from build123d import *

# Parameters (mm, degrees)
BOSS_EXTRUDE1_DEPTH  = 5
SKETCH10_W           = 3
SKETCH10_H           = 3
CUT_EXTRUDE3_DEPTH   = 10
SKETCH11_W           = 10
SKETCH11_H           = 3
CUT_EXTRUDE4_DEPTH   = 10
BOSS_EXTRUDE5_DEPTH  = 3
SKETCH13_R           = 2
BOSS_EXTRUDE6_DEPTH  = 3
SKETCH14_R           = 2
SKETCH14_W           = 7
SKETCH14_H           = 3
BOSS_EXTRUDE7_DEPTH  = 3
SKETCH15_W           = 11.761480784
SKETCH15_H           = 3
BOSS_EXTRUDE8_DEPTH  = 3
SKETCH15_3_W         = 11.761480784
SKETCH15_3_H         = 3
CUT_EXTRUDE6_DEPTH   = 3
CUT_EXTRUDE7_DEPTH   = 63
BOSS_EXTRUDE9_DEPTH  = 3
BOSS_EXTRUDE10_DEPTH = 5
SKETCH19_R           = 2
CUT_EXTRUDE8_DEPTH   = 10
SKETCH24_R           = 1.75
CUT_EXTRUDE12_DEPTH  = 3
BOSS_EXTRUDE12_DEPTH = 3
CUT_EXTRUDE13_DEPTH  = 3
SKETCH27_R           = 2
CUT_EXTRUDE14_DEPTH  = 3
SKETCH29_W           = 25
SKETCH29_H           = 120
BOSS_EXTRUDE13_DEPTH = 1.4
SKETCH30_R           = 2
CUT_EXTRUDE15_DEPTH  = 30.4


with BuildPart() as part:
    # Sketch1 → Boss-Extrude1 (new body)
    with BuildSketch(Plane(origin=(0, 0, 0), x_dir=(1, 0, 0), z_dir=(0, 1, 0))):
        Polygon((-70, -55), (0, -55), (0, 55), (-70, 55), (-85, 40), (-210, 40), (-250, 0), (-210, -40), (-85, -40), align=None)
    extrude(amount=-BOSS_EXTRUDE1_DEPTH)

    # Sketch10 → Cut-Extrude3 (cut)
    with BuildSketch(Plane(origin=(0, 0, 0), x_dir=(1, 0, 0), z_dir=(0, 1, 0))):
        with Locations((-63.236231, -7.5)):
            Rectangle(SKETCH10_W, SKETCH10_H)
        with Locations((-63.236231, -48.5)):
            Rectangle(SKETCH10_W, SKETCH10_H)
        with Locations((-6.5, -48.5)):
            Rectangle(SKETCH10_W, SKETCH10_H)
        with Locations((-6.5, -7.5)):
            Rectangle(SKETCH10_W, SKETCH10_H)
        with Locations((-6.5, 7.5)):
            Rectangle(SKETCH10_W, SKETCH10_H)
        with Locations((-6.5, 48.5)):
            Rectangle(SKETCH10_W, SKETCH10_H)
        with Locations((-63.236231, 48.5)):
            Rectangle(SKETCH10_W, SKETCH10_H)
        with Locations((-63.236231, 7.5)):
            Rectangle(SKETCH10_W, SKETCH10_H)
    extrude(amount=-CUT_EXTRUDE3_DEPTH, mode=Mode.SUBTRACT)

    # Sketch11 → Cut-Extrude4 (cut)
    with BuildSketch(Plane(origin=(0, 0, 0), x_dir=(1, 0, 0), z_dir=(0, 1, 0))):
        with Locations((-13, -35)):
            Rectangle(SKETCH11_W, SKETCH11_H)
        with Locations((-13, 35)):
            Rectangle(SKETCH11_W, SKETCH11_H)
        with Locations((-55, 35)):
            Rectangle(SKETCH11_W, SKETCH11_H)
        with Locations((-55, -35)):
            Rectangle(SKETCH11_W, SKETCH11_H)
    extrude(amount=-CUT_EXTRUDE4_DEPTH, mode=Mode.SUBTRACT)

    # Sketch15<3> → Cut-Extrude6 (cut)
    # profile 1 of 2: a face of its own
    with BuildSketch(Plane(origin=(0, 0, -33.5), x_dir=(-1, 0, 0), z_dir=(0, 0, -1))):
        Polygon((97.670134296, 0), (117.43161508, 0), (117.43161508, 17.663270368), (97.670134296, 22.958343186), align=None)
        Polygon((112.655157945, 10.660908757), (113.43161508, 13.558686236), (106.670134296, 15.370419552), (100.874579339, 16.923333822), (100.098122203, 14.025556343), (105.893677161, 12.472642073), align=None, mode=Mode.SUBTRACT)
    # profile 2 of 2: a face of its own
    with BuildSketch(Plane(origin=(0, 0, -33.5), x_dir=(-1, 0, 0), z_dir=(0, 0, -1))):
        with Locations((107.550874688, -1.5)):
            Rectangle(SKETCH15_3_W, SKETCH15_3_H)
    cut_extrude6 = extrude(amount=CUT_EXTRUDE6_DEPTH, mode=Mode.SUBTRACT)

    # Mirror5: Cut-Extrude6 across plane
    add(cut_extrude6.mirror(Plane.XY), mode=Mode.SUBTRACT)

    # Sketch17 → Cut-Extrude7 (cut)
    with BuildSketch(Plane(origin=(0, 0, 0), x_dir=(1, 0, 0), z_dir=(0, 1, 0))):
        Polygon((-192, -40), (-192, 40), (-210, 40), (-250, 0), (-210, -40), align=None)
    extrude(amount=-CUT_EXTRUDE7_DEPTH, mode=Mode.SUBTRACT)

    # Sketch20 → Boss-Extrude10 (add)
    with BuildSketch(Plane(origin=(0, 0, 0), x_dir=(1, 0, 0), z_dir=(0, 1, 0))):
        Polygon((-115, -40), (-192, -40), (-192, -48), (-123, -48), align=None)
        Polygon((-192, 48), (-192, 40), (-115, 40), (-123, 48), align=None)
    extrude(amount=-BOSS_EXTRUDE10_DEPTH)

    # Sketch19 → Cut-Extrude8 (cut)
    with BuildSketch(Plane(origin=(0, 0, 0), x_dir=(1, 0, 0), z_dir=(0, 1, 0))):
        with Locations(Location((-130.301621673, 11.049999775, 0), (0, 0, 270))):
            Circle(SKETCH19_R)
        with Locations(Location((-178.561621814, 12.319994418, 0), (0, 0, 270))):
            Circle(SKETCH19_R)
        with Locations(Location((-145.541616034, -39.750001917, 0), (0, 0, 270))):
            Circle(SKETCH19_R)
    extrude(amount=-CUT_EXTRUDE8_DEPTH, mode=Mode.SUBTRACT)


with BuildPart() as body_2:
    # Sketch12 → Boss-Extrude5 (new body)
    with BuildSketch(Plane.XY.offset(-36.5)):
        Polygon((-67, 0), (-2, 0), (3.967923412, 30), (15.016198358, 63.505316822), (-12, 56.26634829), (-67, 29.176380902), align=None)
        Polygon((-4.577717242, 39.620171714), (-5.354174377, 42.517949192), (1.407306407, 44.329682508), (2.183763542, 41.431905029), align=None, mode=Mode.SUBTRACT)
    extrude(amount=BOSS_EXTRUDE5_DEPTH)


with BuildPart() as body_3:
    # Mirror3: mirrored copy
    add(body_2.part.mirror(Plane.XY))


with BuildPart() as body_4:
    # Sketch13 → Boss-Extrude6 (new body)
    with BuildSketch(Plane(origin=(-10.211691838, 38.11055277, 0), x_dir=(0.9659258262890699, 0.25881904510251513, 0), z_dir=(-0.25881904510251513, 0.9659258262890699, 0))):
        Polygon((12.8327197, 33.5), (12.8327197, 36.5), (5.8327197, 36.5), (5.8327197, 33.5), (4.8327197, 33.5), (4.8327197, -33.5), (5.8327197, -33.5), (5.8327197, -36.5), (12.8327197, -36.5), (12.8327197, -33.5), (18.8327197, -33.5), (18.8327197, 33.5), align=None)
        with Locations((13.8327197, -25.24)):
            Circle(SKETCH13_R, mode=Mode.SUBTRACT)
        with Locations((13.8327197, 25.24)):
            Circle(SKETCH13_R, mode=Mode.SUBTRACT)
    extrude(amount=BOSS_EXTRUDE6_DEPTH)


with BuildPart() as body_5:
    # Sketch14 → Boss-Extrude7 (new body)
    # profile 1 of 4: a face of its own
    with BuildSketch(Plane(origin=(-10.988148973, 41.008330249, 0), x_dir=(0.9659258262890699, 0.2588190451025152, 0), z_dir=(-0.2588190451025152, 0.9659258262890699, 0))):
        Polygon((-106.0572803, 33.5), (-107.0572803, 33.5), (-107.0572803, 0), (-93.0572803, 0), (-93.0572803, 33.5), (-99.0572803, 33.5), align=None)
        with Locations(Location((-102.0572803, 25.24, 0), (0, 0, 180))):
            Circle(SKETCH14_R, mode=Mode.SUBTRACT)
    # profile 2 of 4: a face of its own
    with BuildSketch(Plane(origin=(-10.988148973, 41.008330249, 0), x_dir=(0.9659258262890699, 0.2588190451025152, 0), z_dir=(-0.2588190451025152, 0.9659258262890699, 0))):
        with Locations((-102.5572803, 35)):
            Rectangle(SKETCH14_W, SKETCH14_H)
    # profile 3 of 4: a face of its own
    with BuildSketch(Plane(origin=(-10.988148973, 41.008330249, 0), x_dir=(0.9659258262890699, 0.2588190451025152, 0), z_dir=(-0.2588190451025152, 0.9659258262890699, 0))):
        Polygon((-93.0572803, 0), (-107.0572803, 0), (-107.0572803, -33.5), (-106.0572803, -33.5), (-99.0572803, -33.5), (-93.0572803, -33.5), align=None)
        with Locations(Location((-102.0572803, -25.24, 0), (0, 0, 180))):
            Circle(SKETCH14_R, mode=Mode.SUBTRACT)
    # profile 4 of 4: a face of its own
    with BuildSketch(Plane(origin=(-10.988148973, 41.008330249, 0), x_dir=(0.9659258262890699, 0.2588190451025152, 0), z_dir=(-0.2588190451025152, 0.9659258262890699, 0))):
        with Locations((-102.5572803, -35)):
            Rectangle(SKETCH14_W, SKETCH14_H)
    extrude(amount=-BOSS_EXTRUDE7_DEPTH)


with BuildPart() as body_6:
    # Sketch15 → Boss-Extrude8 (new body)
    # profile 1 of 3: a face of its own
    with BuildSketch(Plane(origin=(0, 0, -33.5), x_dir=(-1, 0, 0), z_dir=(0, 0, -1))):
        Polygon((97.670134296, 0), (117.43161508, 0), (117.43161508, 17.663270368), (97.670134296, 22.958343186), align=None)
        Polygon((112.655157945, 10.660908757), (113.43161508, 13.558686236), (106.670134296, 15.370419552), (100.874579339, 16.923333822), (100.098122203, 14.025556343), (105.893677161, 12.472642073), align=None, mode=Mode.SUBTRACT)
    # profile 2 of 3: a face of its own
    with BuildSketch(Plane(origin=(0, 0, -33.5), x_dir=(-1, 0, 0), z_dir=(0, 0, -1))):
        with Locations((107.550874688, -1.5)):
            Rectangle(SKETCH15_W, SKETCH15_H)
    # profile 3 of 3: a face of its own
    with BuildSketch(Plane(origin=(0, 0, -33.5), x_dir=(-1, 0, 0), z_dir=(0, 0, -1))):
        Polygon((105.893677161, 12.472642073), (106.670134296, 15.370419552), (100.874579339, 16.923333822), (100.098122203, 14.025556343), align=None)
    extrude(amount=BOSS_EXTRUDE8_DEPTH)


with BuildPart() as body_7:
    # Mirror4: mirrored copy
    add(body_6.part.mirror(Plane.XY))


with BuildPart() as body_8:
    # Sketch18 → Boss-Extrude9 (new body)
    with BuildSketch(Plane(origin=(-12.861561237, -48, 0), x_dir=(0, 0, 1), z_dir=(-0.25881904510252135, -0.9659258262890681, 0))):
        Polygon((48, 185.957758648), (-48, 185.957758648), (-48, 215.180976351), (0, 255.457758648), (48, 215.180976351), align=None)
    extrude(amount=BOSS_EXTRUDE9_DEPTH)

    # Sketch24 → Cut-Extrude12 (cut)
    with BuildSketch(Plane(origin=(-12.861561237, -48, 0), x_dir=(0.9659258262890682, -0.25881904510252135, 0), z_dir=(0.2588190451025213, 0.9659258262890681, 0))):
        with Locations(Location((-200.957758648, -13.875, 0), (0, 0, 180))):
            Circle(SKETCH24_R)
        with Locations(Location((-200.957758648, 13.875, 0), (0, 0, 180))):
            Circle(SKETCH24_R)
    extrude(amount=-CUT_EXTRUDE12_DEPTH, mode=Mode.SUBTRACT)


with BuildPart() as body_9:
    # Sketch26 → Boss-Extrude12 (new body)
    with BuildSketch(Plane.XY.offset(45)):
        Polygon((-172, 3), (-183.927615219, 13.636723728), (-191.439047106, 0), (-185, 0), (-172, 0), align=None)
        Polygon((-210.806452543, 8.145002313), (-211.582909679, 5.247224834), (-199.244443697, 1.941142838), (-192.482962913, 0.129409523), (-193.259420048, -2.768367956), (-200.020900832, -0.956634641), (-212.359366814, 2.349447355), (-213.135823949, -0.548330124), (-196.881901916, -9.881299392), (-192, -1.018389004), (-192, 0), (-191.439047106, 0), (-183.927615219, 13.636723728), align=None)
        Polygon((-192, -1.018389004), (-196.881901916, -9.881299392), (-172, -8), (-172, -5), (-185, -5), (-192, -5), align=None)
        Polygon((-185, 0), (-191.439047106, 0), (-192, -1.018389004), (-192, -5), (-185, -5), align=None)
        Polygon((-192.482962913, 0.129409523), (-199.244443697, 1.941142838), (-200.020900832, -0.956634641), (-193.259420048, -2.768367956), align=None)
        Polygon((-192, -1.018389004), (-191.439047106, 0), (-192, 0), align=None)
    extrude(amount=-BOSS_EXTRUDE12_DEPTH)


with BuildPart() as cut_extrude13_tool:
    # Sketch26<3> → Cut-Extrude13 (new body)
    with BuildSketch(Plane.XY.offset(45)):
        Polygon((-192.482962913, 0.129409523), (-199.244443697, 1.941142838), (-200.020900832, -0.956634641), (-193.259420048, -2.768367956), align=None)
        Polygon((-185, 0), (-191.439047106, 0), (-192, -1.018389004), (-192, -5), (-185, -5), align=None)
        Polygon((-192, -1.018389004), (-191.439047106, 0), (-192, 0), align=None)
    cut_extrude13 = extrude(amount=-CUT_EXTRUDE13_DEPTH)


with BuildPart() as body_8_1:
    add(body_8.part)

    # Cut-Extrude13: cut by cut_extrude13_tool
    add(cut_extrude13_tool.part, mode=Mode.SUBTRACT)


with BuildPart() as part_1:
    add(part.part)

    # Cut-Extrude13: cut by cut_extrude13_tool
    add(cut_extrude13_tool.part, mode=Mode.SUBTRACT)


with BuildPart() as body_10:
    # Mirror7: mirrored copy
    add(body_9.part.mirror(Plane.XY))


with BuildPart() as mirror8_tool:
    # Mirror8: Cut-Extrude13 across plane
    add(cut_extrude13.mirror(Plane.XY))


with BuildPart() as body_8_2:
    add(body_8_1.part)

    # Mirror8: cut by mirror8_tool
    add(mirror8_tool.part, mode=Mode.SUBTRACT)

    # Sketch27 → Cut-Extrude14 (cut)
    with BuildSketch(Plane(origin=(-12.861561237, -48, 0), x_dir=(0.9659258262890681, -0.25881904510252146, 0), z_dir=(0.25881904510252146, 0.9659258262890681, 0))):
        with Locations(Location((-220.731478581, 30.495102239, 0), (0, 0, 180))):
            Circle(SKETCH27_R)
        with Locations(Location((-220.731478581, -30.495102239, 0), (0, 0, 180))):
            Circle(SKETCH27_R)
    extrude(amount=-CUT_EXTRUDE14_DEPTH, mode=Mode.SUBTRACT)


with BuildPart() as part_2:
    add(part_1.part)

    # Mirror8: cut by mirror8_tool
    add(mirror8_tool.part, mode=Mode.SUBTRACT)


with BuildPart() as body_11:
    # Sketch29 → Boss-Extrude13 (new body)
    with BuildSketch(Plane(origin=(-16.226208823, -60.557035742, 0), x_dir=(-0.9659258262890681, 0.25881904510252146, 0), z_dir=(-0.25881904510252146, -0.9659258262890681, 0))):
        with Locations((228.231478581, 0)):
            Rectangle(SKETCH29_W, SKETCH29_H)
    extrude(amount=BOSS_EXTRUDE13_DEPTH)

    # Sketch30 → Cut-Extrude15 (cut)
    with BuildSketch(Plane(origin=(-16.226208823, -60.557035742, 0), x_dir=(0.9659258262890681, -0.2588190451025215, 0), z_dir=(0.2588190451025215, 0.9659258262890681, 0))):
        with Locations(Location((-220.731478581, 30.495102239, 0), (0, 0, 180))):
            Circle(SKETCH30_R)
        with Locations(Location((-220.731478581, -30.495102239, 0), (0, 0, 180))):
            Circle(SKETCH30_R)
    extrude(amount=-CUT_EXTRUDE15_DEPTH, mode=Mode.SUBTRACT)


solid = part_2.part
Read the model definition and answer for the solid it produces. Units are mm, in the model's axes. A direction names the side the tool comes from. Round coordinates to 2 decimals unless told otherwise and drop trailing zeros. Write each loop counter-clockwise with the first axis right and the second up, starting at its lowest first coordinate (ties: lowest second). Pieces come first, ordered by that corner, then holes.
Q1. Find section B-B on y = -0.9. State how many separate pieces and enclosed holes the cut face has, and give its area (3 significant figures).
Values:
separate pieces: 1
enclosed holes: 17
area: 18,500 mm2
Q2. Find section C-C on x = -90.5. Determine the outline of the cut face in (y, z).
Values:
outline: (-5, -40) - (0, -40) - (0, 40) - (-5, 40) - close
Q3. Flat-ended cylindrical pins translate along their axes: P1, Ø2.5, axis at x = -95.5, y = -3, coming from the -Z side; P2, Ø2.5, axis at x = -190, y = -3.5, coming from the -Z side; P3, Ø3, axis at x = -112.5, y = -1, coming from the +Z side. Find the tip coordinate at first contact, or state that the pin passes through.
Values:
P1: stops at z = -40
P2: stops at z = -48
P3: stops at z = 40
Q4. A tool of negligible diameter and unlimited length cuts with its end or side. For faces 4 (the face through (-77, -2, -48)), 5 (the face through (-55, -2, -36.5)), 6 (the face through (-100, -2, 40)), from which of +Z, -Z, +X, -X, +Y, -Y can it reach the whole face along a straight path? Write none if from no direction.
Values:
face 4: -Z, +Y, -Y
face 5: +Y, -Y
face 6: +Z, +Y, -Y
Q5. Find section A-A on x = -158.5. Determine the outline of the cut face in (y, z).
Values:
outline: (-5, -48) - (0, -48) - (0, 48) - (-5, 48) - close
Q6. Straight lines are drawn through the part: line 1 (X direction, y = -2.4, z = -36); line 2 (X direction, y = -3.05, z = -6.5); line 3 (X direction, y = -4.7, z = -35.5). For each, find the intervals that lie inside material, in ascending order.
Values:
line 1: x = -192 to -113.43, -101.67 to -60, -50 to -18, -8 to 0
line 2: x = -192 to -64.74, -61.74 to -8, -5 to 0
line 3: x = -192 to -60, -50 to -18, -8 to 0
Q7. The mould has two halves that part along X. Classify faces 1 (the face through (-78, -2, 47)), 2 (the face through (-189, -2, 42)), 3 (the face through (0, -2, 1)): released by +X, released by -X, zero draft, split by the parting line, or undercut.
Values:
face 1: undercut
face 2: zero draft
face 3: released by +X
